Input: dimensioned drawing with shaded views. Units: mm. Origin: part minimum x, y, z. Give positions to 0.01 mm unless a question says otherwise; leave off trailing zeros. Write each loop counter-clockwise with the first axis right and the second up, starting at its lowest first coordinate (ties: lowest second). Pieces come first, ordered by that corner, then holes. Notation, with made-up numbers: (65.25, -30.75) -> (90.25, -30.75) arc R18 cw to (90.25, -17.75) -> close; hole circle Ø6 at (67, 73.5). An arc over 180 degrees is marked (long way). Answer in a Markdown table with one row per item. Add a question column.
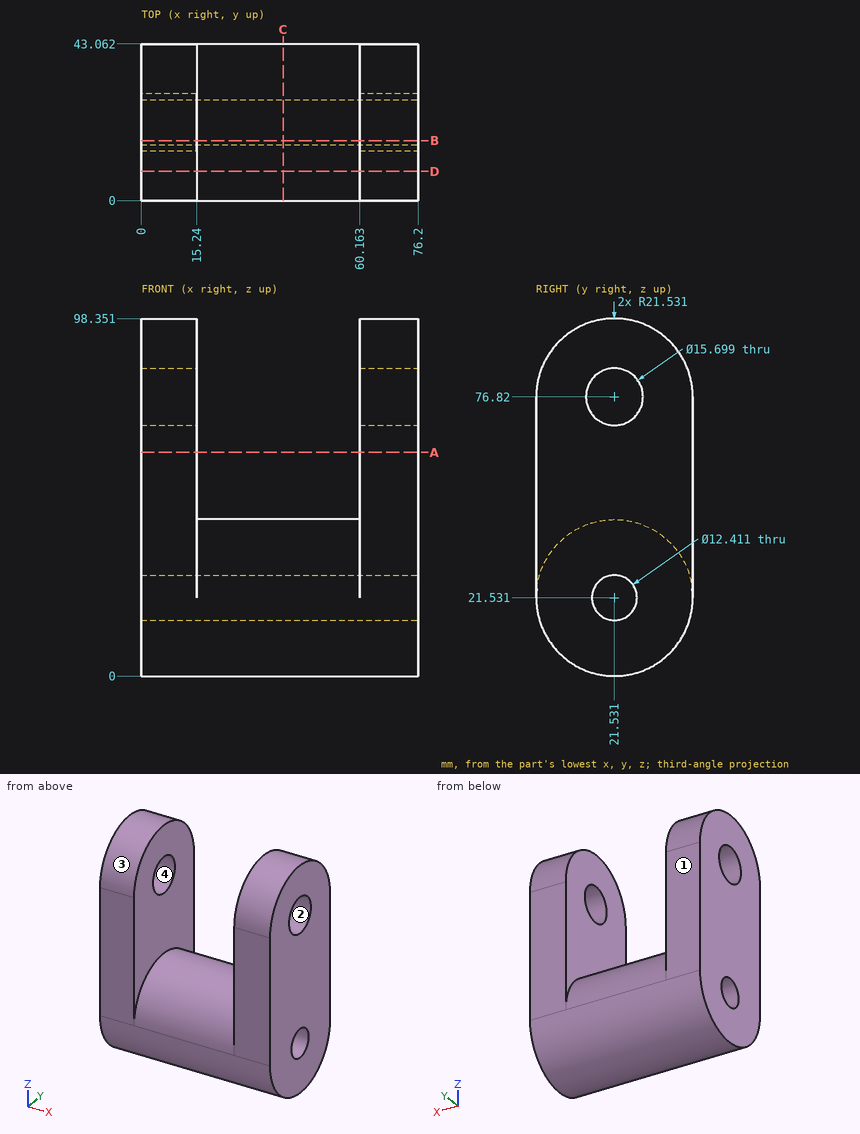
Q1. Section B-B on y = 16.5. Return loops of the section in (x, z) (1 decimal), and give its area (3 significant figures).
Q2. Pull-direction query (Z, two-part tool) for the marked faces 1, 2, 3 and 4; classes: +Z half, -Z half, draft (parallel to the pull), parting line (faces both ways), or undercut.
Q3. Contact query for flat-ended pins moving along their axis: pin 1 Ø10 at (x, z) = (39.5, 10) entering from +Y; pin 2 Ø5 at (x, y) = (32, 34) entering from +Z (1 decimal); pin 3 Ø1 at (x, y) = (47.5, 12.5) entering from +Z. Output: stop coordinate, or through.
Q4. Section C-C on x = 39. Return loops of the section in (y, z) (1 decimal).
Q5. Section A-A on z = 61.5. Return loops of the section in (x, y).
Q6. Line query: probe 1 along X at (y, z) = (3, 64); probe 2 along Y at (x, z) = (31.5, 24) (1 decimal); probe 3 along Z at (x, y) = (51.5, 25) (1 decimal). Output: solid intervals per line, ascending. Write a range as from..to.
Q7. Section D-D on y = 8. Return loops of the section in (x, z), and give its area (3 significant figures).
Checks:
| question | item | result |
|---|---|---|
| 1 | outline | (0, 0.6) -> (76.2, 0.6) -> (76.2, 17.9) -> (0, 17.9) -> close; (0, 25.2) -> (76.2, 25.2) -> (76.2, 70.8) -> (60.2, 70.8) -> (60.2, 42.5) -> (15.2, 42.5) -> (15.2, 70.8) -> (0, 70.8) -> close; (0, 82.8) -> (15.2, 82.8) -> (15.2, 97.8) -> (0, 97.8) -> close; (60.2, 82.8) -> (76.2, 82.8) -> (76.2, 97.8) -> (60.2, 97.8) -> close |
| 1 | area | 3,990 mm^2 |
| 2 | face 1 | draft |
| 2 | face 2 | undercut |
| 2 | face 3 | +Z half |
| 2 | face 4 | undercut |
| 3 | pin 1 | y = 42.05 |
| 3 | pin 2 | z = 40.6 |
| 3 | pin 3 | z = 41.3 |
| 4 | outline | circle Ø43.1 at (21.5, 21.5); hole circle Ø12.4 at (21.5, 21.5) |
| 5 | outline | (0, 0) -> (15.24, 0) -> (15.24, 43.06) -> (0, 43.06) -> close; (60.16, 0) -> (76.2, 0) -> (76.2, 43.06) -> (60.16, 43.06) -> close |
| 6 | probe 1 | 0..15.24, 60.16..76.2 |
| 6 | probe 2 | 0.1..15.8, 27.2..42.9 |
| 6 | probe 3 | 0.3..16.4, 26.7..42.8 |
| 7 | outline | (0, 4.78) -> (76.2, 4.78) -> (76.2, 93.57) -> (60.16, 93.57) -> (60.16, 38.28) -> (15.24, 38.28) -> (15.24, 93.57) -> (0, 93.57) -> close |
| 7 | area | 4,280 mm^2 |
